For this review, use the dimensioned drawing (mm, ordinates from the lowest corner) and the shaded views. Give positions to 0.01 mm unless a question says otherwise; leave off trailing zeros. Write each loop counter-clockwise with the first axis right and the second up, starting at its lowest first coordinate (ties: lowest second). Pieces come first, ordered by that corner, then holes.
1) We need section C-C on z = 7.75. Give the boundary of the cut face in (x, y).
2) For P1, Ø2, axis at x = 6.5, y = 35, coming from the -Z side; P2, Ø4, axis at y = 62, z = 5.5, coming from the +X side; P3, Ø1.5, axis at x = 1, y = 13.5, coming from the -Z side; P4, Ø1, axis at x = 7, y = 56, coming from the +Z side, all flat-tipped, find the tip position at first contact; note any pin that passes through.
3) We need section B-B on x = 8. Give the boundary of the cut face in (y, z), and give its area (3 significant figures).
4) Draft analysis for pull direction X (two halves, no side actions). For the marked faces 1 and 2, state which applies: pulls with the +X half, pulls with the -X half, needs draft (parallel to the pull), parting line crosses it, or undercut.
5) Wall thickness on line 1 along Z through (x, y) = (4.75, 39.5); line 2 along Z through (x, y) = (7.25, 19): over which ranges is each line inside the solid? List them lowest first.
6) We need section A-A on y = 49. Give the boundary of the cut face in (x, z), and give its area (3 significant figures).
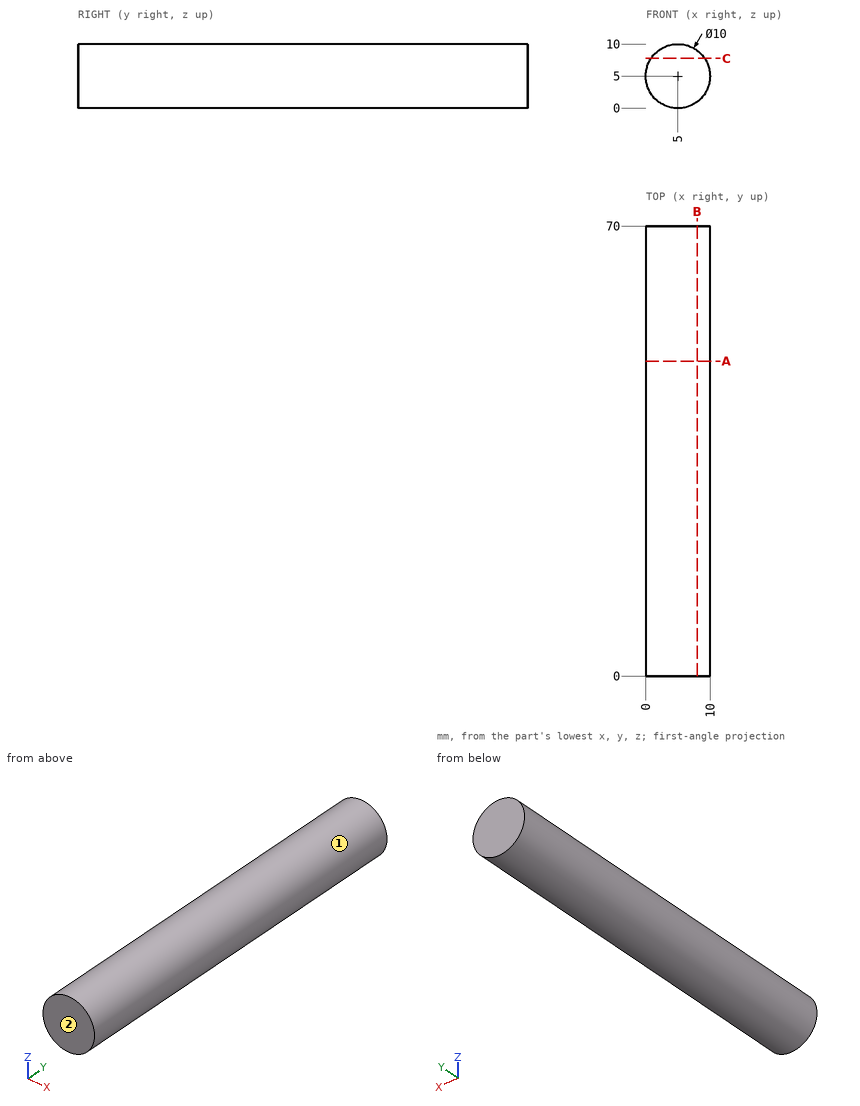
Results list:
1. outline: (0.82, 0) - (9.18, 0) - (9.18, 70) - (0.82, 70) - close
2. P1: stops at z = 0.03
2. P2: stops at x = 10
2. P3: stops at z = 1.2
2. P4: stops at z = 9.77
3. outline: (0, 1) - (70, 1) - (70, 9) - (0, 9) - close
3. area: 560 mm2
4. face 1: parting line crosses it
4. face 2: needs draft
5. line 1: z = 0.01 to 9.99
5. line 2: z = 0.53 to 9.47
6. outline: circle Ø10 at (5, 5)
6. area: 78.5 mm2
